from build123d import *

# Parameters (mm, degrees)
SKETCH1_R           = 9
SKETCH1_W           = 9.1
SKETCH1_H           = 9.1
BOSS_EXTRUDE1_DEPTH = 13
SKETCH2_R           = 9
BOSS_EXTRUDE2_DEPTH = 1
SKETCH3_R           = 5
BOSS_EXTRUDE3_DEPTH = 40
CHAMFER1_SIZE       = 6
SKETCH4_W           = 6
SKETCH4_H           = 4.360376731
CUT_EXTRUDE1_DEPTH  = 34


with BuildPart() as part:
    # Sketch1 → Boss-Extrude1 (new body)
    with BuildSketch(Plane(origin=(0, 0, 0), x_dir=(1, 0, 0), z_dir=(0, 1, 0))):
        with Locations(Location((4.55, 4.55, 0), (0, 0, 90))):
            Circle(SKETCH1_R)
        with Locations((4.55, 4.55)):
            Rectangle(SKETCH1_W, SKETCH1_H, mode=Mode.SUBTRACT)
    extrude(amount=BOSS_EXTRUDE1_DEPTH)

    # Sketch2 → Boss-Extrude2 (add)
    with BuildSketch(Plane(origin=(0, 13, 0), x_dir=(1, 0, 0), z_dir=(0, 1, 0))):
        with Locations(Location((4.55, 4.55, 0), (0, 0, 90))):
            Circle(SKETCH2_R)
    extrude(amount=BOSS_EXTRUDE2_DEPTH)

    # Sketch3 → Boss-Extrude3 (add)
    with BuildSketch(Plane(origin=(0, 14, 0), x_dir=(1, 0, 0), z_dir=(0, 1, 0))):
        with Locations(Location((4.55, 4.443091139, 0), (0, 0, 270))):
            Circle(SKETCH3_R)
    extrude(amount=BOSS_EXTRUDE3_DEPTH)

    # Chamfer1
    # the kernel refuses this chamfer: 6 mm, written as the material it adds along each edge
    with BuildSketch(Plane(origin=(4.55, 14, -4.443091139), x_dir=(0, 0, 1), z_dir=(-1, 0, 0))) as chamfer1_piece_1_section:
        Polygon((5 + CHAMFER1_SIZE, 0), (5, CHAMFER1_SIZE), (5, 0), align=None)
    chamfer1_piece_1 = revolve(axis=Axis((4.55, 14, -4.443091139), (0, 1, 0)), mode=Mode.PRIVATE)
    chamfer1_piece_1 = chamfer1_piece_1 & Plane(origin=(4.55, 17.968075817, -4.55), x_dir=(0, 0, -1), z_dir=(0, -1, 0)) * Cylinder(9, 44, mode=Mode.PRIVATE)
    add(chamfer1_piece_1)

    # Sketch4 → Cut-Extrude1 (cut)
    with BuildSketch(Plane(origin=(0, 54, 0), x_dir=(1, 0, 0), z_dir=(0, 1, 0))):
        Polygon((13.290298635, 2.860978984), (9.514101615, 5.04116735), (6.514101615, -0.154985073), (10.290298635, -2.335173438), align=None)
        with Locations((4.55, 10.623279505)):
            Rectangle(SKETCH4_W, SKETCH4_H)
    extrude(amount=-CUT_EXTRUDE1_DEPTH, mode=Mode.SUBTRACT)


solid = part.part
Model file for the job. Use its own axes, mm. A direction names the side the tool comes from. Give positions to 0.01 mm unless a question says otherwise; leave off trailing zeros. Loops run counter-clockwise (first coordinate to the right, second up) from the corner with the lowest first, then second, coordinate; pieces in that order, holes last.
Item 1: Drop flat-ended pins along their axis: P1, Ø2.5, axis at x = 4.5, z = -3.5, coming from the -Y side; P2, Ø10, axis at x = 6.5, y = 35, coming from the -Z side; P3, Ø3, axis at y = 45, z = -9, coming from the +X side. Give the stop position or say it passes through.
Check values:
P1: stops at y = 13
P2: stops at z = -8.44
P3: stops at x = 8.51
Item 2: Slice it at C-C (y = 17). Write the cut outline in (x, z).
Check values:
outline: circle Ø16 at (4.55, -4.44)
Item 3: Drill centre lines: line 1 along Y through (x, z) = (6.25, -9); line 2 along Z through (x, y) = (2, 9.5); line 3 along Y through (x, z) = (0.5, -7). Where is each one in solid material? Low to high.
Check values:
line 1: y = 13 to 20
line 2: z = -13.18 to -9.1, 0 to 4.08
line 3: y = 13 to 54
Item 4: Slice it at A-A (x = 4.55). Write the cut outline in (y, z), plus the area to 3 significant figures.
Check values:
outline: (0, -13.55) - (15.89, -13.55) - (20, -9.44) - (20, -8.44) - (54, -8.44) - (54, 0.56) - (20, 0.56) - (16.11, 4.45) - (0, 4.45) - (0, 0) - (13, 0) - (13, -9.1) - (0, -9.1) - close
area: 532 mm2
Item 5: Which spindle directions (+Z, -Z, +X, -X, +Y, -Y) get a long thin tool onto all of the face, cutting with end or side? Do faces 4 (the face through (8.894, 36.762, -6.919)), 5 (the face through (5, 37, -8.443)), 6 (the face through (5, 54, -4)), 7 (the face through (4, 6, 0)). Say none if no direction does.
Check values:
face 4: -Z, +X, +Y
face 5: -Z, +X, -X, +Y
face 6: +Z, -Z, +X, -X, +Y
face 7: -Y
Item 6: Slice it at B-B (y = 24.5). Write the cut outline in (x, z), plus the area to 3 significant figures.
Check values:
outline: (1.55, -8.44) - (7.55, -8.44) arc R5 ccw to (9.51, -5.04) - (6.51, 0.15) arc R5 ccw to start
area: 70.4 mm2
Item 7: Mould opens along X. For faces 1 (the face through (8.035, 37.238, -2.479)), 2 (the face through (8, 20, -2)), 3 (the face through (4, 6, -9.1)) say: +X half, -X half, draft (parallel to the pull), parting line (faces both ways), or undercut.
Check values:
face 1: +X half
face 2: draft
face 3: undercut
